Input: part model. Units: mm. Frame: model coordinates. Face numbers are marked on the shaded views. Round coordinates to 2 decimals unless told otherwise and drop trailing zeros. Write each loop counter-clockwise with the first axis right and the second up, starting at its lowest first coordinate (ties: lowest second). Pieces come first, ordered by that corner, then holes. Notation, with made-up numbers: M 77,44 L 116,44 A16 cw 116,53 Z; hole C 46.25,-31.75 d1. An arc over 180 degrees is marked long. Write each question's results on one line, items separated by ' | '. Start each with the question number.
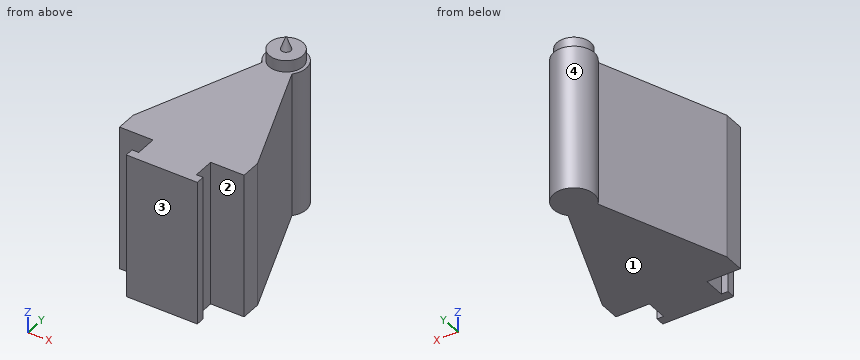
```python
from build123d import *

# Parameters (mm, degrees)
SZKIC1_R                    = 35
DODANIE_WYCI_GNI_CIE2_DEPTH = 250
SZKIC4_R                    = 29.129576732
DODANIE_WYCI_GNI_CIE3_DEPTH = 20
SZKIC5_R                    = 8.316
DODANIE_WYCI_GNI_CIE4_DEPTH = 36
DODANIE_WYCI_GNI_CIE4_TAPER = 20


with BuildPart() as part:
    # Szkic1 → Dodanie-wyciągnięcie2 (new body)
    with BuildSketch(Plane.XY):
        with BuildLine():
            Line((12.5, 179), (12.5, 144))
            Line((12.5, 144), (70.2, 144))
            Line((70.2, 144), (70.2, 107))
            Line((70.2, 107), (58.7, 107))
            Line((58.7, 107), (58.7, 92))
            Line((58.7, 92), (181.3, 92))
            Line((181.3, 92), (181.3, 107))
            Line((181.3, 107), (169.8, 107))
            Line((169.8, 107), (169.8, 144))
            Line((169.8, 144), (227.5, 144))
            Line((227.5, 144), (227.5, 179))
            Line((227.5, 179), (145.832850365, 390.615092801))
            ThreePointArc((145.832850365, 390.615092801), (120, 379.23), (94.167149635, 390.615092801))
            Line((94.167149635, 390.615092801), (12.5, 179))
        make_face()
        with Locations((120, 414.23)):
            Circle(SZKIC1_R)
    extrude(amount=DODANIE_WYCI_GNI_CIE2_DEPTH)

    # Szkic4 → Dodanie-wyciągnięcie3 (add)
    with BuildSketch(Plane.XY.offset(250)):
        with Locations((120, 414.23)):
            Circle(SZKIC4_R)
    extrude(amount=DODANIE_WYCI_GNI_CIE3_DEPTH)

    # Szkic5 → Dodanie-wyciągnięcie4 (add)
    with BuildSketch(Plane.XY.offset(270)):
        with Locations((120, 414.23)):
            Circle(SZKIC5_R)
    extrude(amount=DODANIE_WYCI_GNI_CIE4_DEPTH, taper=DODANIE_WYCI_GNI_CIE4_TAPER)


solid = part.part
```
1. Cut plane A-A on z = 196. Output: boundary loops of the cut face in (x, y), and give its area (3 significant figures).
2. Draft query along Y for the marked faces 1, 2, 3 and 4. Return one class per face: +Y half, -Y half, draft (parallel to the pull), parting line (faces both ways), or undercut.
3. Cut plane B-B on y = 342. Output: boundary loops of the cut face in (x, z), and give its area (3 significant figures).
4. Contact query for flat-ended pins moving along their axis: P1, Ø18.5, axis at y = 130, z = 152.5, coming from the -X side; P2, Ø8, axis at x = 138.5, z = 191, coming from the +Y side; P3, Ø4, axis at y = 320.5, z = 59, coming from the +X side. Output: stop coordinate, or through.
5. Cut plane C-C on x = 214.5. Output: boundary loops of the cut face in (y, z).
6. Line query: L1, parallel to Z at x = 117, y = 228.5; L2, parallel to Z at x = 119.5, y = 396; L3, parallel to X at y = 417, z = 99.5. Output: solid intervals per line, ascending. Write a range as from..to.
Answers follow:
1) outline: M 12.5,144 L 70.2,144 L 70.2,107 L 58.7,107 L 58.7,92 L 181.3,92 L 181.3,107 L 169.8,107 L 169.8,144 L 227.5,144 L 227.5,179 L 145.83,390.62 A35 ccw long 94.17,390.62 L 12.5,179 Z | area: 44,700 mm2
2) face 1: draft | face 2: undercut | face 3: -Y half | face 4: undercut
3) outline: M 75.41,0 L 164.59,0 L 164.59,250 L 75.41,250 Z | area: 22,300 mm2
4) P1: stops at x = 70.2 | P2: stops at y = 446.09 | P3: stops at x = 173.66
5) outline: M 144,0 L 212.69,0 L 212.69,250 L 144,250 Z
6) L1: z = 0..250 | L2: z = 0..270 | L3: x = 85.11..154.89
